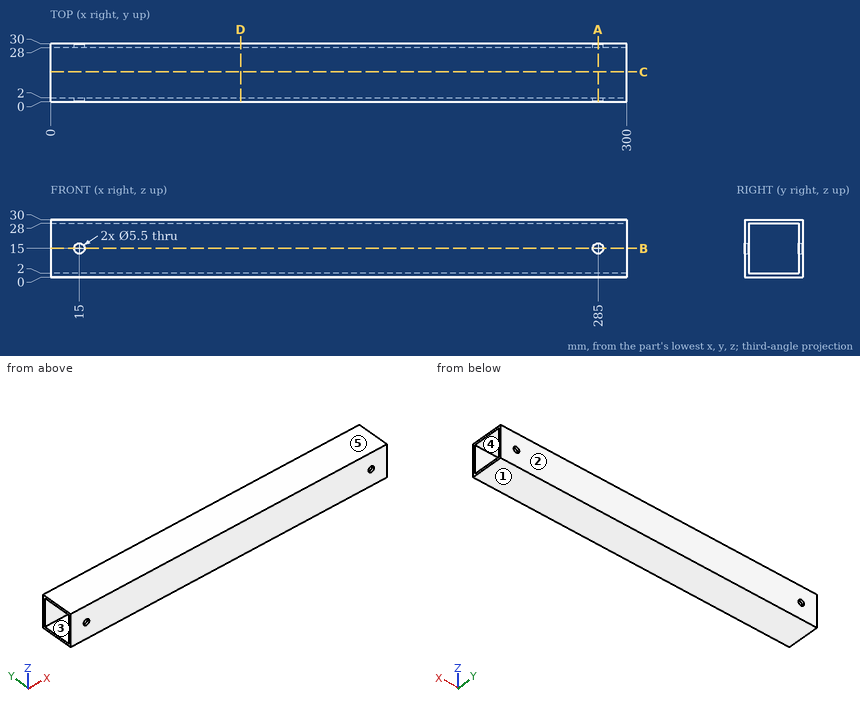
Answer from the drawing. Dimensions are ordinates in mm from the lowest x, y and z of the part. A direction names the side the tool comes from. Coordinates: 2 decimals unless noted, no trailing zeros. Write each loop counter-clockwise with the first axis right and the second up, starting at its lowest first coordinate (ties: lowest second). Pieces come first, ordered by that corner, then holes. Notation, with made-up numbers: M 15,-2.75 L 74,-2.75 A13 cw 74,16.25 Z; hole C -34,-34.75 d4. An arc over 180 degrees is marked long. Use a Markdown table: item, result.
Q1. The part is cut by section D-D, the plane x = 99. Write down the section's boundary in (y, z).
Answer block:
| item | result |
|---|---|
| outline | M 0,0 L 30,0 L 30,30 L 0,30 Z; hole M 2,2 L 28,2 L 28,28 L 2,28 Z |
Q2. The part is cut by section C-C, the plane y = 15.5. Write down the section's boundary in (x, z), then the cut area to 3 significant figures.
Answer block:
| item | result |
|---|---|
| outline | M 0,0 L 300,0 L 300,2 L 0,2 Z; M 0,28 L 300,28 L 300,30 L 0,30 Z |
| area | 1,200 mm2 |
Q3. This flat-tipped pin is pushed along its axis until it touches: pin 1 Ø5 at (x, z) = (15, 15) entering from +Y. Where does it stop, or does it pass through?
Answer block:
| item | result |
|---|---|
| pin 1 | passes through |
Q4. Which of the six approach directions +Z, -Z, +X, -X, +Y, -Y give full straight-line access (tool end or side, diameter ignored) to the marked faces 4 and 5?
Answer block:
| item | result |
|---|---|
| face 4 | +X, -X |
| face 5 | +Z, +X, -X, +Y, -Y |
Q5. The part is cut by section B-B, the plane z = 15. Write down the section's boundary in (x, y), then the cut area to 3 significant figures.
Answer block:
| item | result |
|---|---|
| outline | M 0,0 L 12.25,0 L 12.25,2 L 0,2 Z; M 0,28 L 12.25,28 L 12.25,30 L 0,30 Z; M 17.75,0 L 282.25,0 L 282.25,2 L 17.75,2 Z; M 17.75,28 L 282.25,28 L 282.25,30 L 17.75,30 Z; M 287.75,0 L 300,0 L 300,2 L 287.75,2 Z; M 287.75,28 L 300,28 L 300,30 L 287.75,30 Z |
| area | 1,160 mm2 |
Q6. The part is cut by section A-A, the plane x = 285. Write down the section's boundary in (y, z).
Answer block:
| item | result |
|---|---|
| outline | M 0,0 L 30,0 L 30,12.25 L 28,12.25 L 28,2 L 2,2 L 2,12.25 L 0,12.25 Z; M 0,17.75 L 2,17.75 L 2,28 L 28,28 L 28,17.75 L 30,17.75 L 30,30 L 0,30 Z |
Q7. Straight lines are drawn through the part: L1, parallel to X at y = 28.7, z = 15; L2, parallel to Z at x = 258.5, y = 10.75. For each, find the intervals that lie inside material, in ascending order. Write a range as [from, to].
Answer block:
| item | result |
|---|---|
| L1 | x = [0, 12.25], [17.75, 282.25], [287.75, 300] |
| L2 | z = [0, 2], [28, 30] |
Q8. Determine the mould class of the marked faces 1, 2 and 3 for opening direction Y: released by +Y, released by -Y, zero draft, split by the parting line, or undercut.
Answer block:
| item | result |
|---|---|
| face 1 | zero draft |
| face 2 | released by +Y |
| face 3 | undercut |
